Geometry: final body of the model. Coordinates: model frame, mm. Coordinates: 2 decimals unless noted, no trailing zeros. Write each loop counter-clockwise with the first axis right and the second up, starting at its lowest first coordinate (ties: lowest second). Pieces come first, ordered by that corner, then holes. Notation, with made-up numbers: (1, 78) - (17, 78) arc R26 ccw to (17, 104) - close; hole circle Ø10 at (-26, 18.5). An arc over 180 degrees is marked (long way). Put each result on its own line as item: value.
```python
from build123d import *

# Parameters (mm, degrees)
SKETCH1_W           = 80
SKETCH1_H           = 80
SKETCH1_R           = 5
BOSS_EXTRUDE1_DEPTH = 5
SKETCH2_R           = 14
SKETCH2_R_2         = 7.5
CUT_EXTRUDE1_DEPTH  = 2
CUT_EXTRUDE1_TAPER  = 30
SKETCH3_R           = 2
BOSS_EXTRUDE2_DEPTH = 3


with BuildPart() as part:
    # Sketch1 → Boss-Extrude1 (new body)
    with BuildSketch(Plane.XY):
        Rectangle(SKETCH1_W, SKETCH1_H)
        Circle(SKETCH1_R, mode=Mode.SUBTRACT)
    extrude(amount=BOSS_EXTRUDE1_DEPTH)

    # Sketch2 → Cut-Extrude1 (cut)
    with BuildSketch(Plane.XY.offset(5)):
        Circle(SKETCH2_R)
        Circle(SKETCH2_R_2, mode=Mode.SUBTRACT)
    extrude(amount=-CUT_EXTRUDE1_DEPTH, taper=CUT_EXTRUDE1_TAPER, mode=Mode.SUBTRACT)

    # Sketch3 → Boss-Extrude2 (add)
    with BuildSketch(Plane.XY.offset(5)):
        Polygon((49.67766953, -57.67766953), (14.32233047, -22.32233047), (22.32233047, -14.32233047), (57.67766953, -49.67766953), align=None)
        with Locations((49.497474683, -49.497474683)):
            Circle(SKETCH3_R, mode=Mode.SUBTRACT)
    extrude(amount=BOSS_EXTRUDE2_DEPTH)


solid = part.part
```
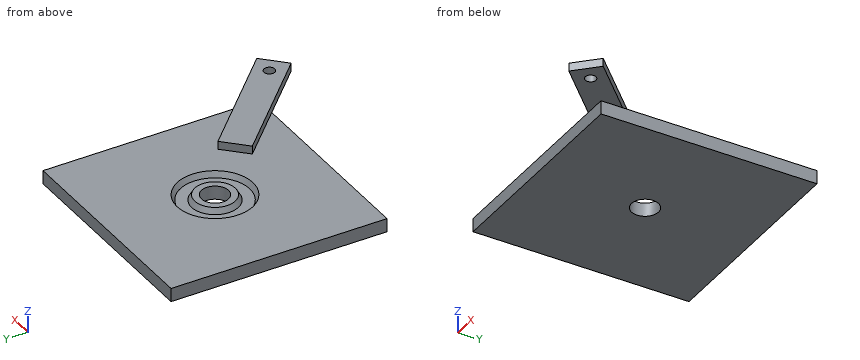
1. Section query C-C (x = 20). Return loops of the section in (y, z).
Answer below:
outline: (-40, 0) - (40, 0) - (40, 5) - (-16.64, 5) - (-16.64, 8) - (-28, 8) - (-28, 5) - (-40, 5) - close
2. Ray query, probe 1 along X at (y, z) = (25, 2); probe 2 along Z at (x, y) = (39.5, 35); probe 3 along X at (y, z) = (-11, 3.75). Return the intervals inside material, ascending. Write a range as from..to.
Answer below:
probe 1: x = -40..40
probe 2: z = 0..5
probe 3: x = -40..-7.44, 7.44..40
3. Section query A-A (x = 0). Return loops of the section in (y, z).
Answer below:
outline: (-40, 0) - (-5, 0) - (-5, 5) - (-7.5, 5) - (-8.65, 3) - (-12.85, 3) - (-14, 5) - (-40, 5) - close; (5, 0) - (40, 0) - (40, 5) - (14, 5) - (12.85, 3) - (8.65, 3) - (7.5, 5) - (5, 5) - close
4. Section query B-B (y = -36). Return loops of the section in (x, z), then the cut area to 3 significant figures.
Answer below:
outline: (-40, 0) - (40, 0) - (40, 5) - (44, 5) - (44, 8) - (28, 8) - (28, 5) - (-40, 5) - close
area: 448 mm²
5. Pin query (flat end, axial travel): pin 1 Ø2.5 at (y, z) = (11.5, 2.5) entering from +X; pin 2 Ø13 at (x, y) = (-4.5, -2.5) entering from +Z; pin 3 Ø13 at (x, y) = (49, -49) entering from -Z. Return the tip coordinate at first contact, or that it passes through.
Answer below:
pin 1: stops at x = 40
pin 2: stops at z = 5
pin 3: stops at z = 5
6. Section query D-D (x = 46). Return loops of the section in (y, z), then the cut area to 3 significant figures.
Answer below:
outline: (-54, 5) - (-38, 5) - (-38, 8) - (-54, 8) - close
area: 48.0 mm²
